Autodesk Inventor part; units mm, degrees
ref_plane "YZ Plane" through (0, 0, 0) normal (1, 0, 0) x (0, 1, 0)
ref_plane "XZ Plane" through (0, 0, 0) normal (0, 1, 0) x (-1, 0, 0)
ref_plane "XY Plane" through (0, 0, 0) normal (0, 0, 1) x (1, 0, 0)
sketch "スケッチ1" plane through (0, 0, 0) normal (0, 1, 0) x (-1, 0, 0)
  line L0 (-10, 8) -> (10, 8)
  line L1 (10, 8) -> (10, -8)
  line L2 (10, -8) -> (-10, -8)
  line L3 (-10, -8) -> (-10, 8)
  line L4 (-10, 8) -> (10, -8) construction
  line L5 (10, 8) -> (-10, -8) construction
  point P0 (0, 0)
  dimension "d0" = 20
  dimension "d1" = 16
extrude "プレート1" add sketch "スケッチ1" along normal blind 2
sketch "スケッチ2" plane through (12, 4, -8) normal (1, 0, 0) x (0, 1, 0)
  line L0 (0, 16) -> (0, 0)
  line L1 (0, 0) -> (21, 0)
  line L2 (21, 0) -> (21, 16)
  line L3 (21, 16) -> (0, 16)
edge flange "フランジ1" height 25 angle 90 thickness 2 bend radius 2 thickness toward (1, 0, 0) relief tear relief width 2 relief depth 1 edges at (10, 2, 0) wall of the first edge with corners at (12, 4, 8) (12, 4, -8) (12, 25, -8) (12, 25, 8)
bend "曲げ1"
corner "コーナー1"
sketch "スケッチ3" plane through (14, 25, 8) normal (1, 0, 0) x (0, 0, -1)
  line L0 (6.5, -4) -> (6.5, -18)
  arc A0 (6.5, -18) -> (9.5, -18) centre (8, -18) ccw
  line L1 (9.5, -18) -> (9.5, -4)
  arc A1 (9.5, -4) -> (6.5, -4) centre (8, -4) ccw
  line L2 (16, 0) -> (16, -21)
  line L3 (0, 0) -> (16, 0)
  point P0 (8, -25)
  point P1 (8, 0)
  dimension "d19" = 1.5
extrude "押し出し1" cut sketch "スケッチ3" against normal blind 10
sketch "スケッチ4" plane through (0, 2, 0) normal (0, 1, 0) x (1, 0, 0)
  line L0 (-6, -1.5) -> (6, -1.5)
  arc A0 (6, -1.5) -> (6, 1.5) centre (6, 0) ccw
  line L1 (6, 1.5) -> (-6, 1.5)
  arc A1 (-6, 1.5) -> (-6, -1.5) centre (-6, 0) ccw
  line L2 (-10, -8) -> (-10, 8)
  line L3 (10, 8) -> (10, -8)
  point P0 (0, 0)
  dimension "d23" = 4
  dimension "d24" = 4
  dimension "d25" = 1.5
extrude "押し出し2" cut sketch "スケッチ4" against normal blind 10
equation "\"d2\" = Thickness"
equation "\"d3\" = BendReliefWidth"
equation "\"d4\" = BendReliefDepth"
equation "\"d5\" = MinimumRemnant"
equation "\"d6\" = TransitionRadius"
equation "\"d9\" = BendRadius"
equation "\"d10\" = CornerReliefSize"
equation "\"d11\" = GapSize"
equation "\"d12\" = JacobiRadiusSize"
equation "\"BendRadius\" = Thickness"
equation "\"BendReliefWidth\" = Thickness"
equation "\"BendReliefDepth\" = 0.5 * Thickness"
equation "\"CornerReliefSize\" = 4 * Thickness"
equation "\"MinimumRemnant\" = 2 * Thickness"
equation "\"TransitionRadius\" = BendRadius"
equation "\"JacobiRadiusSize\" = BendRadius"
equation "\"GapSize\" = Thickness"
properties part number "keyL" material "アルミニウム 6061"
Design review of the part built by this model. Coordinates are the model's own, in mm. A direction names the side the tool comes from. Coordinates: 2 decimals unless noted, no trailing zeros. Write each loop counter-clockwise with the first axis right and the second up, starting at its lowest first coordinate (ties: lowest second). Pieces come first, ordered by that corner, then holes. Notation, with made-up numbers: (-27, 86) - (7, 86) arc R21 cw to (7, 122) - close; hole circle Ø1 at (-33, 40.5). An arc over 180 degrees is marked (long way). One line per item, written item: value.
1) For faces 1 (the face through (12, 14, -2)), 2 (the face through (-7.5, 1, 0)), 3 (the face through (13, 22.5, 0)), 4 (the face through (-10, 1, 0)), 5 (the face through (14, 15, -2)), list the 3-axis set-ups (+Z, -Z, +X, -X, +Y, -Y) from which the entire face can be reached by the end or side of a thin tool; tool diameter is ignored.
Answer sheet:
face 1: +Z, -Z, -X, +Y
face 2: +Y, -Y
face 3: +X, -X
face 4: +Z, -Z, -X, +Y, -Y
face 5: +Z, -Z, +X, +Y, -Y
2) Add section C-C (z = 0). State the section outline as (x, y) points, plus the area to 3 significant figures.
Answer sheet:
outline: (-10, 0) - (-7.5, 0) - (-7.5, 2) - (-10, 2) - close; (7.5, 0) - (10, 0) arc R4 ccw to (14, 4) - (14, 5.5) - (12, 5.5) - (12, 4) arc R2 cw to (10, 2) - (7.5, 2) - close; (12, 22.5) - (14, 22.5) - (14, 25) - (12, 25) - close
area: 27.4 mm2
3) Add section A-A (x = -0.5). State the section outline as (y, z) points.
Answer sheet:
outline: (0, -8) - (2, -8) - (2, -1.5) - (0, -1.5) - close; (0, 1.5) - (2, 1.5) - (2, 8) - (0, 8) - close
4) Add section D-D (z = -3.5). State the section outline as (x, y) points.
Answer sheet:
outline: (-10, 0) - (10, 0) arc R4 ccw to (14, 4) - (14, 25) - (12, 25) - (12, 4) arc R2 cw to (10, 2) - (-10, 2) - close
5) Mouldability with a two-part tool opening along Z and no side actions: class faces 6 (the face through (13, 7, 8)), 7 (the face through (13, 14, -1.5)), 8 (the face through (13, 25, 0)) as +Z half, -Z half, draft (parallel to the pull), parting line (faces both ways), or undercut.
Answer sheet:
face 6: +Z half
face 7: undercut
face 8: draft
6) To check wall thickness, follow probe 1 along Y at (x, z) = (-8.75, 1.25); probe 2 along X at (y, z) = (19.5, 4.75); probe 3 along Z at (x, y) = (12.25, 22.25). State the ranges of each line that lie inside material, in increasing order.
Answer sheet:
probe 1: y = 0 to 2
probe 2: x = 12 to 14
probe 3: z = -8 to -0.83, 0.83 to 8
7) Add section B-B (y = 8). State the section outline as (x, z) points, plus the area to 3 significant figures.
Answer sheet:
outline: (12, -8) - (14, -8) - (14, -1.5) - (12, -1.5) - close; (12, 1.5) - (14, 1.5) - (14, 8) - (12, 8) - close
area: 26.0 mm2
8) Insertion check: pin 1 (1 mm diameter, centred on y = 13.5, z = 2, fed in from -X); pin 2 (8 mm diameter, centred on x = -2, z = -3.5, fed in from +Y); pin 3 (1 mm diameter, centred on y = 3, z = -4, fed in from -X). Each pin has a flat end and moves straight along its axis. Give the tip position at first contact, or say it passes through.
Answer sheet:
pin 1: stops at x = 12
pin 2: stops at y = 2
pin 3: stops at x = 11.32
